Could you check a few things on this model? Use its own coordinates, in mm. Face numbers are marked on the shaded views. A direction names the side the tool comes from. Give positions to 0.01 mm unless a question says otherwise; leave off trailing zeros. Loops run counter-clockwise (first coordinate to the right, second up) from the corner with the lowest first, then second, coordinate; pieces in that order, holes last.
1. I need wall thicknesses on line 1 along Z through (x, y) = (1.5, -3.25); line 2 along X through (y, z) = (-5.25, -0.75); line 3 along X through (y, z) = (-1, 5). Which ranges of each line are inside material? Lowest first, please.
2. Thinking about a two-plate mould opening in Y: for the marked faces 3, 4 and 5, which applies, +Y half, -Y half, draft (parallel to the pull), parting line (faces both ways), or undercut?
3. For the marked faces 1 and 2, which set-ups out of +Z, -Z, +X, -X, +Y, -Y let a thin tool reach every point of the face, with its end or its side?
4. Imagine slicing it at B-B (z = 3.75). List the corners of the cut face in (x, y) for me, plus the area to 3 significant figures.
5. For P1, Ø1, axis at x = 3.5, z = 4, coming from the +Y side; P2, Ø3, axis at x = 2, y = 0.5, coming from the -Z side, each with a flat end and sliding along its axis, tell me the tip position at first contact or that it passes through.
6. Imagine slicing it at A-A (z = -1.25). List the corners of the cut face in (x, y) for me, plus the area to 3 significant figures.
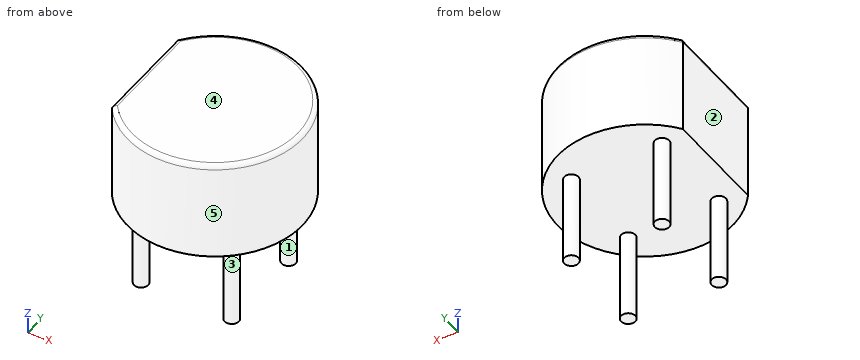
```python
from build123d import *

# Parameters (mm, degrees)
PAD001_DEPTH = 5.6
FILLET_R     = 0.25
SKETCH_R     = 0.4
PAD_DEPTH    = 5


with BuildPart() as fillet_body:
    # Sketch001 → Pad001 (new body)
    with BuildSketch(Plane.XY):
        with BuildLine():
            Line((-1.4, 0.373143), (-1.4, -5.453143))
            ThreePointArc((-1.4, -5.453143), (7.44, -2.54), (-1.4, 0.373143))
        make_face()
    extrude(amount=PAD001_DEPTH)

    # Fillet
    fillet_edges = [fillet_body.edges().sort_by_distance(p)[0] for p in [
        (-1.4, -2.54, 5.6),
        (7.44, -2.54, 5.6),
    ]]
    fillet(fillet_edges, radius=FILLET_R)


with BuildPart() as diode_bridge_round_d9_8mm:
    # Sketch → Pad (new body)
    with BuildSketch(Plane.XY):
        Circle(SKETCH_R)
        with Locations((5.08, 0)):
            Circle(SKETCH_R)
        with Locations((5.08, -5.08)):
            Circle(SKETCH_R)
        with Locations((0, -5.08)):
            Circle(SKETCH_R)
    extrude(amount=-PAD_DEPTH)

    add(fillet_body.part)


solid = diode_bridge_round_d9_8mm.part
```
Derived:
1. line 1: z = 0 to 5.6
1. line 2: x = -0.36 to 0.36, 4.72 to 5.44
1. line 3: x = -1.4 to 7.19
2. face 3: undercut
2. face 4: draft
2. face 5: parting line
3. face 1: -Z
3. face 2: +Z, -Z, -X, +Y, -Y
4. outline: (-1.4, -5.45) arc R4.9 ccw (long way) to (-1.4, 0.37) - close
4. area: 71.6 mm2
5. P1: stops at y = 2.34
5. P2: stops at z = 0
6. outline: circle Ø0.8 at (0, -5.08); circle Ø0.8 at (0, 0); circle Ø0.8 at (5.08, -5.08); circle Ø0.8 at (5.08, 0)
6. area: 2.01 mm2
